Build history of the part. All positions in model axes, mm. A direction names the side the tool comes from. Coordinates: 2 decimals unless noted, no trailing zeros. Order: outer loops, then holes, each group sorted by start corner. A loop starts at its lowest first (then second) coordinate and runs counter-clockwise, first axis right, second up. Notation, with made-up numbers: (-7, 75) - (5, 75) arc R15 cw to (5, 82) - close; hole circle Ø5 at (-22, 10). An arc over 180 degrees is marked (long way). Answer as CSV lines item,"result". Start each with the question number.
Autodesk Fusion 360 part; units mm, degrees
sketch "Sketch1" plane through (0, 0, 0) normal (0, 0, -1) x (1, 0, 0)
  circle A0 centre (10.5, -6.75) radius 1.1
  circle A1 centre (-10.5, -6.75) radius 1.1
  circle A2 centre (10.5, 6.75) radius 1.1
  circle A3 centre (-10.5, 6.75) radius 1.1
  line L0 (12.1, -8.6) -> (12.1, 16.4)
  line L1 (12.1, 16.4) -> (-12.1, 16.4)
  line L2 (-12.1, 16.4) -> (-12.1, -8.6)
  line L3 (-12.1, -8.6) -> (12.1, -8.6)
  line L4 (10, 14.4) -> (-10, 14.4)
  line L5 (-10, 14.4) -> (-10, 11.4)
  line L6 (-10, 11.4) -> (10, 11.4)
  line L7 (10, 11.4) -> (10, 14.4)
  line L8 (10, 14.4) -> (-10, 11.4) construction
  line L9 (-10, 14.4) -> (10, 11.4) construction
  circle A4 centre (0, 0) radius 6
  circle A5 centre (0, 0) radius 7
  line L10 (7.5, 7.5) -> (-7.5, 7.5)
  line L11 (-7.5, 7.5) -> (-7.5, -7.5)
  line L12 (-7.5, -7.5) -> (7.5, -7.5)
  line L13 (7.5, -7.5) -> (7.5, 7.5)
  line L14 (7.5, 7.5) -> (-7.5, -7.5) construction
  line L15 (-7.5, 7.5) -> (7.5, -7.5) construction
  point P0 (0, 12.9)
  dimension "d1" = 20
  dimension "d2" = 3
  dimension "d3" = 15
  dimension "d4" = 15
  dimension "d5" = 12
  dimension "d6" = 14
  dimension "d7" = 2
extrude "Extrude3" add sketch "Sketch1" against normal blind 1 contours L0 L1 L2 L3
extrude "Extrude4" add sketch "Sketch1" against normal blind 3 contours L4 L5 L6 L7
extrude "Extrude5" add sketch "Sketch1" against normal blind 3 contours L10 L11 L12 L13
extrude "Extrude6" add sketch "Sketch1" against normal blind 6 contours A5
extrude "Extrude7" add sketch "Sketch1" against normal blind 19 contours A4
extrude "Extrude8" add sketch "Sketch1" against normal blind 5 from surface at -16 contours A5
(1) Band-saw the part on C-C on z = 12. List the corners of the cut face in (x, y), plus the area to 3 significant figures.
(2) Band-saw the part on D-D on x = 0. List the corners of the cut face in (y, z).
(3) Pull direction Y, two halves, no side cores. Call faces 1 (the flat face through (0, -14.4, 2)), 2 (the flat face through (7.5, 0, 2)), 3 (the cylindrical face through (-9.45, -7.08, 0.49)): +Y half, -Y half, draft (parallel to the pull), parting line (faces both ways), or undercut.
(4) Drop flat-ended pins along their axis: pin 1 Ø0.6 at (x, z) = (1.5, 1.5) entering from -Y; pin 2 Ø2.5 at (x, y) = (-10.5, 6.75) entering from +Z; pin 3 Ø5 at (x, z) = (-7.5, 18) entering from -Y. Give the stop position or say it passes through.
(5) Band-saw the part on A-A on x = -10.5. List the corners of the cut face in (y, z), plus the area to 3 significant figures.
(6) Probe L1, parallel to Y at x = -10.5, z = 0.6; L2, parallel to X at y = 6.75, z = 0.8; L3, parallel to X at y = 0, z = 19.8. List the from-to ranges inside material, lowest first. Write a range as [from, to].
(7) Which spindle directions (+Z, -Z, +X, -X, +Y, -Y) get a long thin tool onto all of the face, cutting with end or side? Do faces 4 (the flat face through (0, 7.5, 2)), 5 (the flat face through (0, -13, 3)), 6 (the flat face through (0, 0, 19)), 7 (the cylindrical face through (-6, 0, 11)), 8 (the flat face through (10, -13, 2)). Say none if no direction does.
(8) Band-saw the part on B-B on y = -13.5. List the corners of the cut face in (x, z).
Filled in:
1,outline,"circle Ø12 at (0, 0)"
1,area,"113 mm^2"
2,outline,"(-16.4, 0) - (8.6, 0) - (8.6, 1) - (7.5, 1) - (7.5, 3) - (7, 3) - (7, 6) - (6, 6) - (6, 16) - (7, 16) - (7, 21) - (6, 21) - (6, 19) - (-6, 19) - (-6, 21) - (-7, 21) - (-7, 16) - (-6, 16) - (-6, 6) - (-7, 6) - (-7, 3) - (-7.5, 3) - (-7.5, 1) - (-11.4, 1) - (-11.4, 3) - (-14.4, 3) - (-14.4, 1) - (-16.4, 1) - close"
3,face 1,"-Y half"
3,face 2,"draft"
3,face 3,"undercut"
4,pin 1,"stops at y = -14.4"
4,pin 2,"stops at z = 1"
4,pin 3,"stops at y = -4.9"
5,outline,"(-16.4, 0) - (-7.85, 0) - (-7.85, 1) - (-16.4, 1) - close; (-5.65, 0) - (5.65, 0) - (5.65, 1) - (-5.65, 1) - close; (7.85, 0) - (8.6, 0) - (8.6, 1) - (7.85, 1) - close"
5,area,"20.6 mm^2"
6,L1,"y = [-16.4, -7.85], [-5.65, 5.65], [7.85, 8.6]"
6,L2,"x = [-12.1, -11.6], [-9.4, 9.4], [11.6, 12.1]"
6,L3,"x = [-7, -6], [6, 7]"
7,face 4,"+Z, +X, -X, +Y"
7,face 5,"+Z, +X, -X, -Y"
7,face 6,"+Z"
7,face 7,"none"
7,face 8,"+Z, +X, +Y, -Y"
8,outline,"(-12.1, 0) - (12.1, 0) - (12.1, 1) - (10, 1) - (10, 3) - (-10, 3) - (-10, 1) - (-12.1, 1) - close"
